```python
from build123d import *

# Parameters (mm, degrees)
SKETCH4_W           = 50
SKETCH4_H           = 40
BOSS_EXTRUDE1_DEPTH = 5
SKETCH5_R           = 2.25
BOSS_EXTRUDE2_DEPTH = 11.26
SKETCH6_W           = 50
SKETCH6_H           = 5
BOSS_EXTRUDE3_DEPTH = 5


with BuildPart() as part:
    # Sketch3 → Revolve1 (revolve)
    with BuildSketch(Plane.XY, mode=Mode.PRIVATE) as revolve1_sk:
        Polygon((0, 0), (10, 0), (10, 8.26), (7.5, 8.26), (7.5, 11.26), (0, 11.26), align=None)
    revolve(revolve1_sk.sketch.rotate(Axis((0, 11.26, 0), (0, -1, 0)), 180), axis=Axis((0, 11.26, 0), (0, -1, 0)))

    # Sketch4 → Boss-Extrude1 (add)
    with BuildSketch(Plane.XZ):
        Rectangle(SKETCH4_W, SKETCH4_H)
    extrude(amount=BOSS_EXTRUDE1_DEPTH)

    # Sketch5 → Boss-Extrude2 (add)
    with BuildSketch(Plane(origin=(0, 0, 0), x_dir=(1, 0, 0), z_dir=(0, 1, 0))):
        with Locations((-16, 0)):
            Circle(SKETCH5_R)
    extrude(amount=BOSS_EXTRUDE2_DEPTH)

    # Sketch6 → Boss-Extrude3 (add)
    with BuildSketch(Plane(origin=(0, 0, -20), x_dir=(-1, 0, 0), z_dir=(0, 0, -1))):
        with Locations((0, -2.5)):
            Rectangle(SKETCH6_W, SKETCH6_H)
    extrude(amount=BOSS_EXTRUDE3_DEPTH)


solid = part.part
```
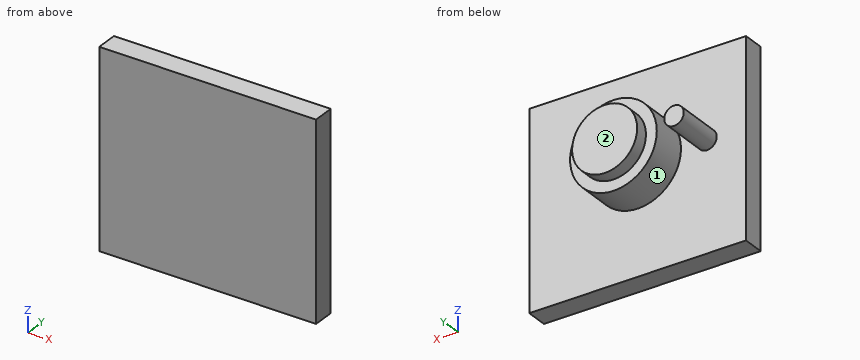
The model under review builds one solid part; all positions refer to its coordinate system, in mm. Face numbers are marked on the shaded views. A direction names the side the tool comes from. Coordinates: 2 decimals unless noted, no trailing zeros. Order: outer loops, then holes, each group sorted by start corner. A loop starts at its lowest first (then second) coordinate and runs counter-clockwise, first axis right, second up. Notation, with made-up numbers: (82.5, -17.5) -> (135.5, -17.5) arc R21 cw to (135.5, 21.5) -> close; hole circle Ø4 at (57, 37.25). An arc over 180 degrees is marked (long way). Answer in a Markdown table with one row per item. Add a question column.
Item 1: We need section C-C on x = 0. Write out the cut boundary in (y, z).
Item 2: Machinability: for the marked faces 1 and 2, which of the approach directions +Z, -Z, +X, -X, +Y, -Y give a long, thin tool a straight path to every point of the face, cutting with its end or side? Answer none if there is none.
Item 3: We need section A-A on z = 0. Write out the cut boundary in (x, y).
Item 4: Clearance check with flat-ended pins moving along their axes: pin 1 (4 mm diameter, centred on y = 5, z = 10.5, fed in from -X); pin 2 (3 mm diameter, centred on x = 7, y = 6, fed in from -Z). State where each tip first meets the part, or that it passes through.
Item 5: We need section B-B on y = 4.75. Write out the cut boundary in (x, z), plus the area to 3 significant figures.
Item 6: To check wall thickness, follow probe 1 along Y at (x, z) = (-10, -21.5); probe 2 along X at (y, z) = (4, 1); probe 3 along X at (y, z) = (1.25, 3). State the ranges of each line that lie inside material, in increasing order.
Item 7: We need section D-D on x = 5. Write out the cut boundary in (y, z), plus the area to 3 significant figures.
Final values:
| question | item | result |
|---|---|---|
| 1 | outline | (-5, -25) -> (0, -25) -> (0, -10) -> (8.26, -10) -> (8.26, -7.5) -> (11.26, -7.5) -> (11.26, 7.5) -> (8.26, 7.5) -> (8.26, 10) -> (0, 10) -> (0, 20) -> (-5, 20) -> close |
| 2 | face 1 | +Y |
| 2 | face 2 | +Z, -Z, +X, -X, +Y |
| 3 | outline | (-25, -5) -> (25, -5) -> (25, 0) -> (10, 0) -> (10, 8.26) -> (7.5, 8.26) -> (7.5, 11.26) -> (-7.5, 11.26) -> (-7.5, 8.26) -> (-10, 8.26) -> (-10, 0) -> (-13.75, 0) -> (-13.75, 11.26) -> (-18.25, 11.26) -> (-18.25, 0) -> (-25, 0) -> close |
| 4 | pin 1 | stops at x = -5.27 |
| 4 | pin 2 | stops at z = -8.35 |
| 5 | outline | circle Ø4.5 at (-16, 0); circle Ø20 at (0, 0) |
| 5 | area | 330 mm2 |
| 6 | probe 1 | y = -5 to 0 |
| 6 | probe 2 | x = -18.02 to -13.98, -9.95 to 9.95 |
| 6 | probe 3 | x = -9.54 to 9.54 |
| 7 | outline | (-5, -25) -> (0, -25) -> (0, -8.66) -> (8.26, -8.66) -> (8.26, -5.59) -> (11.26, -5.59) -> (11.26, 5.59) -> (8.26, 5.59) -> (8.26, 8.66) -> (0, 8.66) -> (0, 20) -> (-5, 20) -> close |
| 7 | area | 402 mm2 |
